Check sheet for the modelled part. Datum: model origin and axes. Units: mm. A direction names the side the tool comes from. Round coordinates to 2 decimals unless told otherwise and drop trailing zeros. Loops run counter-clockwise (first coordinate to the right, second up) from the corner with the lowest first, then second, coordinate; pieces in that order, holes last. Notation, with made-up numbers: (-8.5, -28) - (41.5, -28) arc R12 cw to (41.5, -5) - close; hole circle Ø2 at (66.25, 3.5). An arc over 180 degrees is marked (long way). Return JSON: item names as keys, results as strings.
from build123d import *

# Parameters (mm, degrees)
ESQUISSE1_W             = 62
ESQUISSE1_H             = 8
BOSS_EXTRU_1_DEPTH      = 55
ESQUISSE2_R             = 15
ESQUISSE2_R_2           = 13
ENL_V_MAT_EXTRU_1_DEPTH = 5
ESQUISSE3_R             = 1.5
ENL_V_MAT_EXTRU_2_DEPTH = 10
ESQUISSE4_R             = 1.5
ENL_V_MAT_EXTRU_3_DEPTH = 10
ESQUISSE5_R             = 1.5
ENL_V_MAT_EXTRU_4_DEPTH = 56
ESQUISSE6_R             = 5
ENL_V_MAT_EXTRU_5_DEPTH = 9


with BuildPart() as part:
    # Esquisse1 → Boss.-Extru.1 (new body)
    with BuildSketch(Plane.XY):
        with Locations((25.5, -49)):
            Rectangle(ESQUISSE1_W, ESQUISSE1_H)
    extrude(amount=BOSS_EXTRU_1_DEPTH)

    # Esquisse2 → Enlèv. mat.-Extru.1 (cut)
    with BuildSketch(Plane(origin=(0, -45, 0), x_dir=(-1, 0, 0), z_dir=(0, 1, 0))):
        with Locations((-25.5, 27.5)):
            Circle(ESQUISSE2_R)
        with Locations((-25.5, 27.5)):
            Circle(ESQUISSE2_R_2, mode=Mode.SUBTRACT)
    extrude(amount=-ENL_V_MAT_EXTRU_1_DEPTH, mode=Mode.SUBTRACT)

    # Esquisse3 → Enlèv. mat.-Extru.2 (cut)
    with BuildSketch(Plane.ZY.offset(5.5)):
        with Locations((12.5, -47.5)):
            Circle(ESQUISSE3_R)
        with Locations((42.5, -47.5)):
            Circle(ESQUISSE3_R)
    extrude(amount=-ENL_V_MAT_EXTRU_2_DEPTH, mode=Mode.SUBTRACT)

    # Esquisse4 → Enlèv. mat.-Extru.3 (cut)
    with BuildSketch(Plane(origin=(56.5, 0, 0), x_dir=(0, 0, -1), z_dir=(1, 0, 0))):
        with Locations((-42.5, -47.5)):
            Circle(ESQUISSE4_R)
        with Locations((-12.5, -47.5)):
            Circle(ESQUISSE4_R)
    extrude(amount=-ENL_V_MAT_EXTRU_3_DEPTH, mode=Mode.SUBTRACT)

    # Esquisse5 → Enlèv. mat.-Extru.4 (cut, through all)
    with BuildSketch(Plane(origin=(0, 0, 0), x_dir=(-1, 0, 0), z_dir=(0, 0, -1))):
        with Locations((-25.5, -47.5)):
            Circle(ESQUISSE5_R)
    extrude(amount=-ENL_V_MAT_EXTRU_4_DEPTH, mode=Mode.SUBTRACT)

    # Esquisse6 → Enlèv. mat.-Extru.5 (cut, through all)
    with BuildSketch(Plane(origin=(0, -45, 0), x_dir=(1, 0, 0), z_dir=(0, 1, 0))):
        with Locations((25.5, -27.5)):
            Circle(ESQUISSE6_R)
    extrude(amount=-ENL_V_MAT_EXTRU_5_DEPTH, mode=Mode.SUBTRACT)


solid = part.part
Q1. Draft check along Z on faces 6 (the face through (25, -53, 21)), 7 (the face through (4.5, -47, 42)), 8 (the face through (25, -50, 0)). Enter one of: released by +Z, released by -Z, zero draft, split by the parting line, or undercut.
Answer key:
{"face 6": "zero draft", "face 7": "undercut", "face 8": "released by -Z"}
Q2. Depth check by flat-ended pin: P1, Ø1.5, axis at y = -47.5, z = 42, coming from the -X side; P2, Ø0.9, axis at y = -47, z = 12, coming from the +X side. Enter the tip coordinate at first touch or a pass-through.
Answer key:
{"P1": "stops at x = 4.5", "P2": "stops at x = 46.5"}
Q3. Sectioned sample at B-B (x = -1). Enter the section's corners in (y, z), plus the area to 3 significant figures.
Answer key:
{"outline": "(-53, 0) - (-45, 0) - (-45, 55) - (-53, 55) - close; hole circle Ø3 at (-47.5, 12.5); hole circle Ø3 at (-47.5, 42.5)", "area": "426 mm²"}
Q4. Sectioned sample at D-D (y = -47.5). State how many separate pieces and enclosed holes the cut face has, plus the area to 3 significant figures.
Answer key:
{"separate pieces": "4", "enclosed holes": "0", "area": "2,910 mm²"}
Q5. Sectioned sample at A-A (z = 27.5). Enter the section's corners in (x, y), plus the area to 3 significant figures.
Answer key:
{"outline": "(-5.5, -53) - (20.5, -53) - (20.5, -45) - (12.5, -45) - (12.5, -50) - (10.5, -50) - (10.5, -45) - (-5.5, -45) - close; (30.5, -53) - (56.5, -53) - (56.5, -45) - (40.5, -45) - (40.5, -50) - (38.5, -50) - (38.5, -45) - (30.5, -45) - close", "area": "396 mm²"}
Q6. Scan lines: probe 1 along Y at (x, z) = (25.5, 47.25); probe 2 along Z at (x, y) = (-1, -48); probe 3 along Z at (x, y) = (31.5, -47). Record each from-to range of solid material in increasing order. Write a range as [from, to].
Answer key:
{"probe 1": "y = [-53, -49], [-46, -45]", "probe 2": "z = [0, 11.09], [13.91, 41.09], [43.91, 55]", "probe 3": "z = [0, 13.75], [15.97, 39.03], [41.25, 55]"}
Q7. Tool access check on faces 1 (the face through (18.51, -47.46, 38.46)), 2 (the face through (31, -45, 27)), 3 (the face through (-0.6, -48.4, 41.3)), 4 (the face through (46.5, -47, 13)), 5 (the face through (25.825, -48.964, 48.623)). Record the directions out of +Z, -Z, +X, -X, +Y, -Y that give a thin tool (end or side, any length) a straight path to the whole face; none if there is none.
Answer key:
{"face 1": "+Y", "face 2": "+Z, -Z, +X, -X, +Y", "face 3": "-X", "face 4": "+X", "face 5": "+Z, -Z"}
Q8. Sectioned sample at C-C (z = 39.5). Enter the section's corners in (x, y).
Answer key:
{"outline": "(-5.5, -53) - (56.5, -53) - (56.5, -45) - (34.5, -45) - (34.5, -50) - (30.5, -50) - (30.5, -45) - (20.5, -45) - (20.5, -50) - (16.5, -50) - (16.5, -45) - (-5.5, -45) - close; hole circle Ø3 at (25.5, -47.5)"}
